Geometry: final body of the model. Coordinates: model frame, mm. A direction names the side the tool comes from. Give positions to 0.01 mm unless a question says otherwise; leave off trailing zeros. Write each loop counter-clockwise with the first axis right and the second up, starting at its lowest first coordinate (ties: lowest second). Pieces come first, ordered by that corner, then holes. Notation, with made-up numbers: M 24.5,-26.5 L 56.5,-26.5 A29 cw 56.5,10.5 Z; hole C 4,79 d3. An arc over 180 degrees is marked long. Use a Markdown table: item, result. Add a question column.
(1) Draft query along X for faces 1 (the flat face through (-7, 30.814, 18)), 2 (the flat face through (30, 0, 68.072)), 3 (the flat face through (-41.125, -1, 34)). Return one class per face: released by +X, released by -X, zero draft, split by the parting line, or undercut.
(2) Cut plane A-A (x = -28.5). Output: boundary loops of the cut face in (y, z).
(3) Cut plane C-C (y = -14). Output: boundary loops of the cut face in (x, z), plus the area to 3 significant figures.
(4) Material intervals for L1, parallel to X at y = 4, z = 14; L2, parallel to X at y = -26, z = 57; L3, parallel to Y at x = -6.5, z = 13.5, sorted ascending.
(5) Cut plane D-D (z = 28). Output: boundary loops of the cut face in (x, y), plus the area to 3 significant figures.
(6) Cut plane B-B (z = 42). Output: boundary loops of the cut face in (x, y), plus the area to 3 significant figures.
(7) Reachability of faces 4 (the flat face through (34.549, -1, 34)), 5 (the flat face through (-25.4, 32, 51)), 6 (the flat face through (19.605, 7, 16)) from +Z, -Z, +X, -X, +Y, -Y: full face, straight path, thin tool, end or side. Return the list, or none.
```python
from build123d import *

# Parameters (mm, degrees)
F0_W     = 75.673942
F0_H     = 68.772793
F1_DEPTH = 68.072
F2_W     = 53.099798
F2_H     = 46.344617
F3_DEPTH = 104.902
F4_W     = 137.758225
F4_H     = 67.900397
F5_DEPTH = 25.4


with BuildPart() as f1:
    # F0 (on Top) → F1 (new body)
    with BuildSketch(Plane.XY):
        with Locations((-3.288293, -0.885312)):
            Rectangle(F0_W, F0_H)
    extrude(amount=F1_DEPTH)

    # F2 (on Top) → F3 (cut)
    with BuildSketch(Plane.XY):
        with Locations((-6.945002, 7.641886)):
            Rectangle(F2_W, F2_H)
    extrude(amount=F3_DEPTH, mode=Mode.SUBTRACT)

    # F4 (on Right) → F5 (cut, symmetric)
    with BuildSketch(Plane.YZ):
        with Locations((14.477775, 66.976663)):
            Rectangle(F4_W, F4_H)
    extrude(amount=F5_DEPTH, both=True, mode=Mode.SUBTRACT)


solid = f1.part
```
Answer list:
| question | item | result |
|---|---|---|
| 1 | face 1 | undercut |
| 1 | face 2 | zero draft |
| 1 | face 3 | released by -X |
| 2 | outline | M -35.27,0 L -15.53,0 L -15.53,68.07 L -35.27,68.07 Z; M 30.81,0 L 33.5,0 L 33.5,68.07 L 30.81,68.07 Z |
| 3 | outline | M -41.13,0 L -33.49,0 L -33.49,68.07 L -41.13,68.07 Z; M 19.6,0 L 34.55,0 L 34.55,68.07 L 25.4,68.07 L 25.4,33.03 L 19.6,33.03 Z |
| 3 | area | 1,330 mm² |
| 4 | L1 | -41.13 to -33.49, 19.6 to 34.55 |
| 4 | L2 | -41.13 to -25.4, 25.4 to 34.55 |
| 4 | L3 | -35.27 to -15.53, 30.81 to 33.5 |
| 5 | outline | M -41.13,-35.27 L 34.55,-35.27 L 34.55,33.5 L -41.13,33.5 Z; hole M -33.49,-15.53 L 19.6,-15.53 L 19.6,30.81 L -33.49,30.81 Z |
| 5 | area | 2,740 mm² |
| 6 | outline | M -41.13,-35.27 L -25.4,-35.27 L -25.4,-15.53 L -33.49,-15.53 L -33.49,30.81 L -25.4,30.81 L -25.4,33.5 L -41.13,33.5 Z; M 25.4,-35.27 L 34.55,-35.27 L 34.55,33.5 L 25.4,33.5 Z |
| 6 | area | 1,340 mm² |
| 7 | face 4 | +Z, -Z, +X, +Y, -Y |
| 7 | face 5 | +Z, +Y, -Y |
| 7 | face 6 | +Z, -Z |
